Can you work these out from the model? Positions are in its coordinate system, mm. A direction names the side the tool comes from. Coordinates: 2 decimals unless noted, no trailing zeros. Write each loop counter-clockwise with the first axis right and the second up, starting at its lowest first coordinate (ties: lowest second). Pieces come first, ordered by that corner, then holes. Notation, with made-up numbers: (37.25, 58.25) -> (85.25, 58.25) arc R22 ccw to (85.25, 90.25) -> close; hole circle Ø6 at (84, -12). An arc over 180 degrees is marked (long way). Use one line per item in the form item = value.
```python
from build123d import *

# Parameters (mm, degrees)
SKETCH1_W           = 88.9
SKETCH1_H           = 44.45
SKETCH1_R           = 3.323105079
BOSS_EXTRUDE1_DEPTH = 101.6
SKETCH2_R           = 3.175
SKETCH2_W           = 42.3
SKETCH2_H           = 42.3
CUT_EXTRUDE1_DEPTH  = 120.474537036


with BuildPart() as part:
    # Sketch1 → Boss-Extrude1 (new body)
    with BuildSketch(Plane(origin=(0, 0, 0), x_dir=(1, 0, 0), z_dir=(0, 1, 0))):
        Rectangle(SKETCH1_W, SKETCH1_H)
        with Locations(Location((0, 0, 0), (0, 0, 270))):
            Circle(SKETCH1_R, mode=Mode.SUBTRACT)
    extrude(amount=BOSS_EXTRUDE1_DEPTH)

    # Sketch2 → Cut-Extrude1 (cut, through all)
    with BuildSketch(Plane.XY.offset(22.225)):
        with Locations((0, 85.09)):
            Circle(SKETCH2_R)
        with Locations((0, 33.85)):
            Rectangle(SKETCH2_W, SKETCH2_H)
    extrude(amount=-CUT_EXTRUDE1_DEPTH, mode=Mode.SUBTRACT)


solid = part.part
```
Q1. Suppose I cut it at C-C (z = -17). Write out the boundary of the cut face in (x, y) (3 decimals).
Return value:
outline = (-44.45, 0) -> (44.45, 0) -> (44.45, 101.6) -> (-44.45, 101.6) -> close; hole (-21.15, 12.7) -> (21.15, 12.7) -> (21.15, 55) -> (-21.15, 55) -> close; hole circle Ø6.35 at (0, 85.09)
Q2. If I drill on line 1 (Y direction, x = 0, z = -7.5) (3 decimals); line 2 (Y direction, x = 20.5, z = 14.5); line 3 (X direction, y = 85, z = 11), over which ranges is the centre line in solid material (lowest first)? Write a range as from..to.
Return value:
line_1 = 0..12.7, 55..81.915, 88.265..101.6
line_2 = 0..12.7, 55..101.6
line_3 = -44.45..-3.17, 3.17..44.45
Q3. Suppose I cut it at A-A (y = 16.5). Write out the boundary of the cut face in (x, z) (3 decimals), then the cut area to 3 significant figures.
Return value:
outline = (-44.45, -22.225) -> (-21.15, -22.225) -> (-21.15, 22.225) -> (-44.45, 22.225) -> close; (21.15, -22.225) -> (44.45, -22.225) -> (44.45, 22.225) -> (21.15, 22.225) -> close
area = 2,070 mm2
Q4. Will these pins go through, and if not, where does the flat tip stop? pin 1 (4 mm diameter, centred on x = 0, z = 0, fed in from +Y); pin 2 (10.5 mm diameter, centred on x = 0, z = 0, fed in from -Y).
Return value:
pin_1 = through
pin_2 = 0
Q5. Thinking about a two-plate mould opening in Y: for faces 1 (the flat face through (-5, 12.7, 0)), 2 (the flat face through (-1, 0, -5)), 3 (the flat face through (-1, 101.6, -5)), 4 (the cylindrical face through (-1.27, 77.97, 3.07)), which applies, released by +Y, released by -Y, zero draft, split by the parting line, or undercut?
Return value:
face_1 = undercut
face_2 = released by -Y
face_3 = released by +Y
face_4 = zero draft
Q6. Suppose I cut it at B-B (x = 0). Write out the boundary of the cut face in (y, z) (3 decimals).
Return value:
outline = (0, -22.225) -> (12.7, -22.225) -> (12.7, -3.323) -> (0, -3.323) -> close; (0, 3.323) -> (12.7, 3.323) -> (12.7, 22.225) -> (0, 22.225) -> close; (55, -22.225) -> (81.915, -22.225) -> (81.915, -3.323) -> (55, -3.323) -> close; (55, 3.323) -> (81.915, 3.323) -> (81.915, 22.225) -> (55, 22.225) -> close; (88.265, -22.225) -> (101.6, -22.225) -> (101.6, -3.323) -> (88.265, -3.323) -> close; (88.265, 3.323) -> (101.6, 3.323) -> (101.6, 22.225) -> (88.265, 22.225) -> close
Q7. Suppose I cut it at D-D (y = 85.09). Write out the boundary of the cut face in (x, z) (3 decimals).
Return value:
outline = (-44.45, -22.225) -> (-3.175, -22.225) -> (-3.175, -0.981) arc R3.323 cw to (-3.175, 0.981) -> (-3.175, 22.225) -> (-44.45, 22.225) -> close; (3.175, -22.225) -> (44.45, -22.225) -> (44.45, 22.225) -> (3.175, 22.225) -> (3.175, 0.981) arc R3.323 cw to (3.175, -0.981) -> close
Q8. For faces 5 (the flat face through (-44.45, 50, 0)), 6 (the flat face through (21.15, 34, 0)), which set-ups out of +Z, -Z, +X, -X, +Y, -Y let a thin tool reach every point of the face, with its end or its side?
Return value:
face_5 = +Z, -Z, -X, +Y, -Y
face_6 = +Z, -Z
